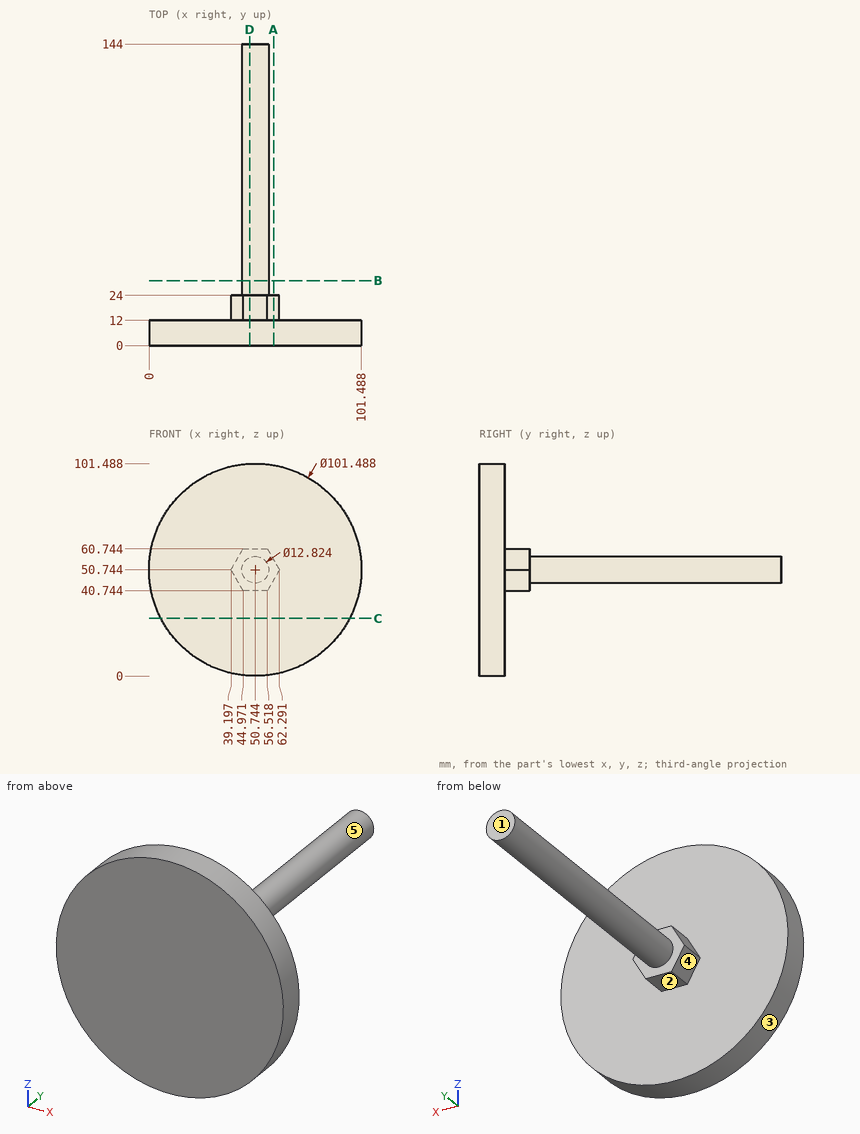
Verification items for this drawing (mm, ordinates from the low corner). A direction names the side the tool comes from. Round coordinates to 2 decimals unless told otherwise and drop trailing zeros. Order: outer loops, then holes, each group sorted by start corner. A loop starts at its lowest first (then second) coordinate and runs counter-clockwise, first axis right, second up.
1) Material ranges on line 1 (Y direction, x = 33, z = 46.5); line 2 (Z direction, x = 51, y = 106); line 3 (X direction, y = 71, z = 56.5) (1 decimal), recorded low to high.
Geometry says:
line 1: y = 0 to 12
line 2: z = 44.34 to 57.15
line 3: x = 47.9 to 53.6
2) Tool access check on the marked faces 1, 2, 3, 4 and 5. Record the directions out of +Z, -Z, +X, -X, +Y, -Y that give a thin tool (end or side, any length) a straight path to the whole face; none if there is none.
Geometry says:
face 1: +Z, -Z, +X, -X, +Y
face 2: -Z, +X, -X, +Y
face 3: +Y, -Y
face 4: -Z, -X, +Y
face 5: +Y
3) Depth check by flat-ended pin: pin 1 (8 mm diameter, centred on x = 37.5, z = 28, fed in from +Y); pin 2 (12.5 mm diameter, centred on x = 51, y = 20, fed in from -Z); pin 3 (4 mm diameter, centred on y = 116, z = 58, fed in from -X). Enter the tip coordinate at first touch or a pass-through.
Geometry says:
pin 1: stops at y = 12
pin 2: stops at z = 40.74
pin 3: stops at x = 47.07
4) Cross-section at C-C, the plane z = 27.5. Record the cut outline in (x, y).
Geometry says:
outline: (5.64, 0) - (95.85, 0) - (95.85, 12) - (5.64, 12) - close
5) Cross-section at A-A, the plane x = 59.5. Record the cut outline in (y, z).
Geometry says:
outline: (0, 0.76) - (12, 0.76) - (12, 45.91) - (24, 45.91) - (24, 55.58) - (12, 55.58) - (12, 100.73) - (0, 100.73) - close
6) Cross-section at B-B, the plane y = 31. Record the cut outline in (x, z) (1 decimal), plus the area to 3 significant figures.
Geometry says:
outline: circle Ø12.8 at (50.7, 50.7)
area: 129 mm2
7) Cross-section at D-D, the plane x = 48. Record the cut outline in (y, z) (1 decimal), plus the area to 3 significant figures.
Geometry says:
outline: (0, 0.1) - (12, 0.1) - (12, 40.7) - (24, 40.7) - (24, 44.9) - (144, 44.9) - (144, 56.5) - (24, 56.5) - (24, 60.7) - (12, 60.7) - (12, 101.4) - (0, 101.4) - close
area: 2,850 mm2
